from build123d import *

# Parameters (mm, degrees)
ESTRUSIONE_ESTRUSIONE1_DEPTH = 20
SCHIZZO2_W                   = 4
SCHIZZO2_H                   = 4
TAGLIO_ESTRUSIONE2_DEPTH     = 20
SCHIZZO3_W                   = 10
SCHIZZO3_H                   = 6.102364877
ESTRUSIONE_ESTRUSIONE3_DEPTH = 2
ESTRUSIONE_ESTRUSIONE4_DEPTH = 1.6
ESTRUSIONE_ESTRUSIONE5_DEPTH = 1.6
SCHIZZO15_W                  = 10
SCHIZZO15_H                  = 2
ESTRUSIONE_ESTRUSIONE6_DEPTH = 8.5
ESTRUSIONE_ESTRUSIONE7_DEPTH = 1.6
ESTRUSIONE_ESTRUSIONE8_DEPTH = 1.6
SCHIZZO24_W                  = 10
SCHIZZO24_H                  = 2
ESTRUSIONE_ESTRUSIONE9_DEPTH = 8.5
RACCORDO1_RADIUS             = 5
RACCORDO1_LENGTH             = 2
RACCORDO2_RADIUS             = 5
RACCORDO2_LENGTH             = 2
RACCORDO3_R                  = 4
RACCORDO4_R                  = 4
RACCORDO6_R                  = 2
SCHIZZO28_R                  = 1.4
TAGLIO_ESTRUSIONE5_DEPTH     = 10
SCHIZZO29_R                  = 1.4
TAGLIO_ESTRUSIONE6_DEPTH     = 10


with BuildPart() as part:
    # Schizzo1 → Estrusione-Estrusione1 (new body)
    with BuildSketch(Plane(origin=(0, 0, 0), x_dir=(1, 0, 0), z_dir=(0, 1, 0))):
        Polygon((-16, 0), (0, 0), (33, -10.5), (53, -10.5), (85.612492158, 0), (101.612492158, 0), (101.612492158, -10.5), (111.612492158, -10.5), (111.612492158, -8.5), (103.612492158, -8.5), (103.612492158, 2), (85.29846697, 2), (52.685974812, -8.5), (33.310512217, -8.5), (0.310512217, 2), (-18, 2), (-18, -8.5), (-26, -8.5), (-26, -10.5), (-16, -10.5), align=None)
    extrude(amount=ESTRUSIONE_ESTRUSIONE1_DEPTH)

    # Schizzo2 → Taglio-Estrusione2 (cut)
    with BuildSketch(Plane.XY):
        with Locations((-11.5, 16)):
            Rectangle(SCHIZZO2_W, SCHIZZO2_H)
        with Locations((-4.5, 16)):
            Rectangle(SCHIZZO2_W, SCHIZZO2_H)
        with Locations((-4.5, 10)):
            Rectangle(SCHIZZO2_W, SCHIZZO2_H)
        with Locations((-4.5, 4)):
            Rectangle(SCHIZZO2_W, SCHIZZO2_H)
        with Locations((-11.5, 10)):
            Rectangle(SCHIZZO2_W, SCHIZZO2_H)
        with Locations((-11.5, 4)):
            Rectangle(SCHIZZO2_W, SCHIZZO2_H)
        with Locations((97.5, 4)):
            Rectangle(SCHIZZO2_W, SCHIZZO2_H)
        with Locations((90.5, 4)):
            Rectangle(SCHIZZO2_W, SCHIZZO2_H)
        with Locations((90.5, 10)):
            Rectangle(SCHIZZO2_W, SCHIZZO2_H)
        with Locations((97.5, 10)):
            Rectangle(SCHIZZO2_W, SCHIZZO2_H)
        with Locations((90.5, 16)):
            Rectangle(SCHIZZO2_W, SCHIZZO2_H)
        with Locations((97.5, 16)):
            Rectangle(SCHIZZO2_W, SCHIZZO2_H)
    extrude(amount=-TAGLIO_ESTRUSIONE2_DEPTH, mode=Mode.SUBTRACT)

    # Schizzo3 → Estrusione-Estrusione3 (add)
    with BuildSketch(Plane.XY.offset(10.5)):
        with Locations((43, 23.051182438)):
            Rectangle(SCHIZZO3_W, SCHIZZO3_H)
        with Locations((43, -3.051182439)):
            Rectangle(SCHIZZO3_W, SCHIZZO3_H)
    extrude(amount=-ESTRUSIONE_ESTRUSIONE3_DEPTH)

    # Schizzo4 → Estrusione-Estrusione4 (add)
    with BuildSketch(Plane.XZ):
        Polygon((-16, 0), (-16, 10.5), (33, 10.5), (0, 0), align=None)
    extrude(amount=-ESTRUSIONE_ESTRUSIONE4_DEPTH)

    # Schizzo6 → Estrusione-Estrusione5 (add)
    with BuildSketch(Plane.XZ):
        Polygon((101.612492158, 10.5), (53, 10.5), (85.612492158, 0), (101.612492158, 0), align=None)
    extrude(amount=-ESTRUSIONE_ESTRUSIONE5_DEPTH)

    # Schizzo15 → Estrusione-Estrusione6 (add)
    with BuildSketch(Plane.XY.offset(10.5)):
        with Locations((43, 1)):
            Rectangle(SCHIZZO15_W, SCHIZZO15_H)
    extrude(amount=ESTRUSIONE_ESTRUSIONE6_DEPTH)

    # Schizzo20 → Estrusione-Estrusione7 (add)
    with BuildSketch(Plane(origin=(0, 20, 0), x_dir=(1, 0, 0), z_dir=(0, 1, 0))):
        Polygon((101.612492158, -10.5), (53, -10.5), (85.612492158, 0), (101.612492158, 0), align=None)
    extrude(amount=-ESTRUSIONE_ESTRUSIONE7_DEPTH)

    # Schizzo23 → Estrusione-Estrusione8 (add)
    with BuildSketch(Plane(origin=(0, 20, 0), x_dir=(1, 0, 0), z_dir=(0, 1, 0))):
        Polygon((-16, -10.5), (33, -10.5), (0, 0), (-16, 0), align=None)
    extrude(amount=-ESTRUSIONE_ESTRUSIONE8_DEPTH)

    # Schizzo24 → Estrusione-Estrusione9 (add)
    with BuildSketch(Plane.XY.offset(10.5)):
        with Locations((43, 19)):
            Rectangle(SCHIZZO24_W, SCHIZZO24_H)
    extrude(amount=ESTRUSIONE_ESTRUSIONE9_DEPTH)

    # Raccordo1: full round fillet: the end face becomes a half cylinder, R = half its width
    raccordo1_face = Plane((43, 19, 19), x_dir=(0, -1, 0), z_dir=(0, 0, 1))  # on the end face: x along it, z out of the body
    raccordo1_slab = raccordo1_face.offset(-RACCORDO1_RADIUS / 2) * Box(RACCORDO1_LENGTH, 2 * RACCORDO1_RADIUS, RACCORDO1_RADIUS, mode=Mode.PRIVATE)  # the body's end, R deep
    raccordo1_round = Plane((43, 19, 14), x_dir=(0, 0, 1), z_dir=(0, -1, 0)) * Cylinder(RACCORDO1_RADIUS, RACCORDO1_LENGTH, mode=Mode.PRIVATE)  # its axis R under the face
    add(raccordo1_slab - raccordo1_round, mode=Mode.SUBTRACT)

    # Raccordo2: full round fillet: the end face becomes a half cylinder, R = half its width
    raccordo2_face = Plane((43, 1, 19), x_dir=(0, 1, 0), z_dir=(0, 0, 1))  # on the end face: x along it, z out of the body
    raccordo2_slab = raccordo2_face.offset(-RACCORDO2_RADIUS / 2) * Box(RACCORDO2_LENGTH, 2 * RACCORDO2_RADIUS, RACCORDO2_RADIUS, mode=Mode.PRIVATE)  # the body's end, R deep
    raccordo2_round = Plane((43, 1, 14), x_dir=(0, 0, 1), z_dir=(0, 1, 0)) * Cylinder(RACCORDO2_RADIUS, RACCORDO2_LENGTH, mode=Mode.PRIVATE)  # its axis R under the face
    add(raccordo2_slab - raccordo2_round, mode=Mode.SUBTRACT)

    # Raccordo3
    # the kernel refuses this fillet: 4 mm, written as the material it adds along each edge
    with BuildSketch(Plane(origin=(48, 2, 10.5), x_dir=(1, 0, 0), z_dir=(0, -1, 0)), Plane(origin=(38, 0, 10.5), x_dir=(-1, 0, 0), z_dir=(0, 1, 0)), Plane(origin=(38, 18, 10.5), x_dir=(-1, 0, 0), z_dir=(0, 1, 0)), Plane(origin=(48, 20, 10.5), x_dir=(1, 0, 0), z_dir=(0, -1, 0))) as raccordo3_piece_1:
        with BuildLine():
            CenterArc((3.986100378, 4), RACCORDO3_R, 183.184738537, 86.815261463)
            Line((-0.007722012, 3.777777778), (-0.407104251, 3.755555556))
            ThreePointArc((-0.407104251, 3.755555556), (-0.4, 3.5), (-0.4, 0))
            Line((-0.4, 0), (0, -0.4))
            Line((0, -0.4), (3.986100378, -0.4))
            Line((3.986100378, -0.4), (3.986100378, 0))
        make_face()
    extrude(amount=2)
    # the kernel refuses this fillet: 4 mm, written as the material it takes off along each edge
    with BuildSketch(Plane(origin=(-26, 0, -1.5), x_dir=(0, 1, 0), z_dir=(0, 0, 1)), Plane(origin=(111.612492158, 0, 20.5), x_dir=(0, 1, 0), z_dir=(0, 0, -1))) as raccordo3_2_piece_1:
        with BuildLine():
            CenterArc((RACCORDO3_R, -RACCORDO3_R), RACCORDO3_R, 90, 90)
            Line((0, -RACCORDO3_R), (0, 0))
            Line((0, 0), (RACCORDO3_R, 0))
        make_face()
    extrude(amount=22, mode=Mode.SUBTRACT)
    with BuildSketch(Plane(origin=(111.612492158, 20, 20.5), x_dir=(0, -1, 0), z_dir=(0, 0, -1)), Plane(origin=(-26, 20, -1.5), x_dir=(0, -1, 0), z_dir=(0, 0, 1))) as raccordo3_2_piece_2:
        with BuildLine():
            CenterArc((RACCORDO3_R, RACCORDO3_R), RACCORDO3_R, 180, 90)
            Line((0, RACCORDO3_R), (0, 0))
            Line((0, 0), (RACCORDO3_R, 0))
        make_face()
    extrude(amount=22, mode=Mode.SUBTRACT)

    # Raccordo4
    # the kernel refuses this fillet: 4 mm, written as the material it adds along each edge
    with BuildSketch(Plane(origin=(48, 20, 8.5), x_dir=(1, 0, 0), z_dir=(0, 0, 1)), Plane(origin=(38, 20, 10.5), x_dir=(-1, 0, 0), z_dir=(0, 0, -1)), Plane(origin=(38, 0, 8.5), x_dir=(-1, 0, 0), z_dir=(0, 0, 1)), Plane(origin=(48, 0, 10.5), x_dir=(1, 0, 0), z_dir=(0, 0, -1))) as raccordo4_piece_1:
        with BuildLine():
            CenterArc((RACCORDO4_R, RACCORDO4_R), RACCORDO4_R, 180, 90)
            Line((0, RACCORDO4_R), (0, 0))
            Line((0, 0), (RACCORDO4_R, 0))
        make_face()
    extrude(amount=2)

    # Raccordo6
    raccordo6_edges = [part.edges().sort_by_distance(p)[0] for p in [
        (38, 26.102364877, 9.5),
        (48, 26.102364877, 9.5),
        (48, -6.102364877, 9.5),
        (38, -6.102364877, 9.5),
    ]]
    fillet(raccordo6_edges, radius=RACCORDO6_R)

    # Schizzo28 → Taglio-Estrusione5 (cut)
    with BuildSketch(Plane(origin=(42.230610684, 213.6, 10.5), x_dir=(1, 0, 0), z_dir=(0, 0, 1))):
        with Locations((0.769389316, -189.997635123)):
            Circle(SCHIZZO28_R)
        with Locations((0.769389316, -217.202364877)):
            Circle(SCHIZZO28_R)
    extrude(amount=-TAGLIO_ESTRUSIONE5_DEPTH, mode=Mode.SUBTRACT)

    # Schizzo29 → Taglio-Estrusione6 (cut)
    with BuildSketch(Plane(origin=(42.230610684, 213.6, 10.5), x_dir=(1, 0, 0), z_dir=(0, 0, 1))):
        with Locations((-65.730610684, -203.6)):
            Circle(SCHIZZO29_R)
        with Locations((67.269389316, -203.6)):
            Circle(SCHIZZO29_R)
    extrude(amount=-TAGLIO_ESTRUSIONE6_DEPTH, mode=Mode.SUBTRACT)


solid = part.part
CAD build for the part. Positions are in the model's coordinates, mm. A direction names the side the tool comes from. Coordinates: 2 decimals unless noted, no trailing zeros. Order: outer loops, then holes, each group sorted by start corner. A loop starts at its lowest first (then second) coordinate and runs counter-clockwise, first axis right, second up. Notation, with made-up numbers: (35.25, 49.25) -> (83.25, 49.25) arc R26 cw to (83.25, 75.25) -> close; hole circle Ø5 at (-32.5, 82). An arc over 180 degrees is marked (long way). Answer in a Markdown table with one row per item.
1) Which spindle directions (+Z, -Z, +X, -X, +Y, -Y) get a long thin tool onto all of the face, cutting with end or side? Do faces 1 (the face through (107.7, 9.9, 8.5)), 2 (the face through (69.078, 9.882, 5.323)), 3 (the face through (43, 10, 8.5)), 4 (the face through (0, 0, 6)), 5 (the face through (80, 0, 6)). Say none if no direction does.
Check values:
| item | result |
|---|---|
| face 1 | -Z, +X, +Y, -Y |
| face 2 | +Z |
| face 3 | -Z, +Y, -Y |
| face 4 | +Z, -Z, -X, -Y |
| face 5 | +Z, -Z, +X, -Y |
2) Flat gauge pins, fed straight in: P1, Ø5, axis at x = 97, y = 9, coming from the +Z side; P2, Ø3.5, axis at x = 43, y = 23.6, coming from the -Z side; P3, Ø12, axis at x = 88, y = 12, coming from the +Z side. Where does each tip first touch, or does it go through?
Check values:
| item | result |
|---|---|
| P1 | z = 0 |
| P2 | z = 8.5 |
| P3 | z = 1.16 |
3) Mould opens along X. For faces 6 (the face through (-24.797, 18.859, 9.486)), 7 (the face through (101.612, 10, 5)), 8 (the face through (-9, 10, -2)) say: pulls with the +X half, pulls with the -X half, needs draft (parallel to the pull), parting line crosses it, or undercut.
Check values:
| item | result |
|---|---|
| face 6 | pulls with the -X half |
| face 7 | undercut |
| face 8 | needs draft |
4) Band-saw the part on C-C (x = 109.5). List the corners of the cut face in (y, z).
Check values:
| item | result |
|---|---|
| outline | (0.47, 8.5) -> (8.6, 8.5) -> (8.6, 10.5) -> (0.47, 10.5) -> close; (11.4, 8.5) -> (19.53, 8.5) -> (19.53, 10.5) -> (11.4, 10.5) -> close |
5) Drill centre lines: line 1 (Y direction, x = 43, z = 10.1); line 2 (Y direction, x = 20, z = 8.75); line 3 (Y direction, x = 109.5, z = 8.9). Where is each one in solid material? Low to high.
Check values:
| item | result |
|---|---|
| line 1 | -6.1 to -5, -2.2 to 22.2, 25 to 26.1 |
| line 2 | 0 to 1.6, 18.4 to 20 |
| line 3 | 0.47 to 8.6, 11.4 to 19.53 |
6) Band-saw the part on B-B (z = 17.5). List the corners of the cut face in (x, y), and give its area (3 significant figures).
Check values:
| item | result |
|---|---|
| outline | (39.43, 0) -> (46.57, 0) -> (46.57, 2) -> (39.43, 2) -> close; (39.43, 18) -> (46.57, 18) -> (46.57, 20) -> (39.43, 20) -> close |
| area | 28.6 mm2 |
7) Band-saw the part on D-D (y = 10). Give the number of separate pieces and of enclosed holes in the cut face, and give its area (3 significant figures).
Check values:
| item | result |
|---|---|
| separate pieces | 7 |
| enclosed holes | 0 |
| area | 281 mm2 |
8) Band-saw the part on A-A (z = 5.5). List the corners of the cut face in (x, y), and give its area (3 significant figures).
Check values:
| item | result |
|---|---|
| outline | (-18, 0) -> (23.88, 0) -> (23.88, 20) -> (-18, 20) -> close; (62, 0) -> (103.61, 0) -> (103.61, 20) -> (62, 20) -> close; hole (-16, 1.6) -> (17.29, 1.6) -> (17.29, 18.4) -> (-16, 18.4) -> close; hole (68.53, 1.6) -> (101.61, 1.6) -> (101.61, 18.4) -> (68.53, 18.4) -> close |
| area | 555 mm2 |
